Autodesk Inventor part; units mm, degrees
ref_plane "YZ Plane" through (0, 0, 0) normal (1, 0, 0) x (0, 1, 0)
ref_plane "XZ Plane" through (0, 0, 0) normal (0, 1, 0) x (-1, 0, 0)
ref_plane "XY Plane" through (0, 0, 0) normal (0, 0, 1) x (1, 0, 0)
sketch "スケッチ1" plane through (0, 0, 0) normal (0, 0, 1) x (1, 0, 0)
  circle A0 centre (0, 0) radius 21
  dimension "d0" = 42
extrude "押し出し1" add sketch "スケッチ1" along normal blind 5
sketch "スケッチ2" plane through (0, 0, 5) normal (0, 0, 1) x (1, 0, 0)
  circle A0 centre (0, 0) radius 14
  circle A1 centre (0, 0) radius 17.5
  circle A2 centre (0, 0) radius 21
  dimension "d3" = 28
  dimension "d8" = 7
  dimension "d9" = 3.5
extrude "押し出し3" add sketch "スケッチ2" along normal blind 5 contours A1
fillet "フィレット1" radius 1 4 edges at (-14, 0, 10) (-17.5, 0, 10) (-17.5, 0, 5) (-21, 0, 5)
extrude "押し出し4" add sketch "スケッチ2" along normal blind 4 contours A0
equation "\"d9\" = 0.5 * d8"
properties part number "inkpad"
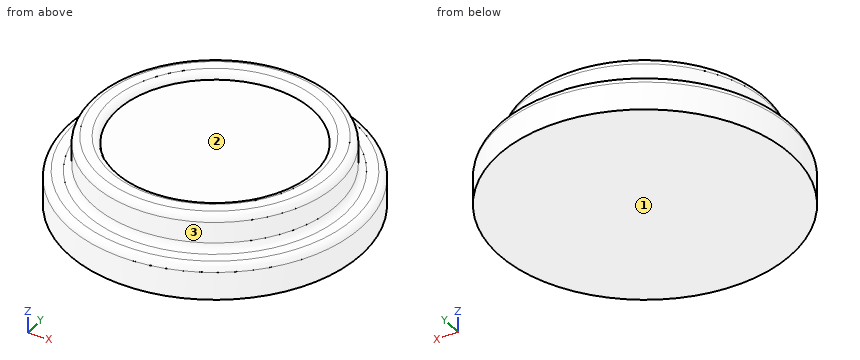
The listing builds one solid part. Answer for the finished solid, in the listing's coordinates (mm). Face numbers are marked on the shaded views. Round coordinates to 2 decimals unless told otherwise and drop trailing zeros. Loops run counter-clockwise (first coordinate to the right, second up) from the corner with the lowest first, then second, coordinate; pieces in that order, holes last. Notation, with made-up numbers: (-24, -15) -> (25, -15) arc R27 cw to (25, 16) -> close; hole circle Ø4 at (51, -13). An arc over 180 degrees is marked (long way). Use one line per item in the form item = value.
1. The part is cut by section C-C on z = 1.5. Determine the outline of the cut face in (x, y).
Answer key:
outline = circle Ø42 at (0, 0)
2. Find the intervals of material crossed by probe 1 along Z at (x, y) = (8, 2); probe 2 along Y at (x, z) = (-4.5, 6.75); probe 3 along X at (y, z) = (3.5, 7.5), in increasing order. Write a range as [from, to].
Answer key:
probe_1 = [0, 9]
probe_2 = [-16.91, 16.91]
probe_3 = [-17.15, 17.15]
3. For a pull along Y with two mould halves and no side action, classify the marked faces 1, 2 and 3 as released by +Y, released by -Y, zero draft, split by the parting line, or undercut.
Answer key:
face_1 = zero draft
face_2 = undercut
face_3 = split by the parting line
4. Flat-ended cylindrical pins translate along their axes: pin 1 Ø12 at (x, y) = (4, 0) entering from +Z; pin 2 Ø22.5 at (x, y) = (3.5, 0) entering from +Z; pin 3 Ø1.5 at (y, z) = (9.5, 3) entering from +X. Find the tip coordinate at first contact, or state that the pin passes through.
Answer key:
pin_1 = 9
pin_2 = 9.97
pin_3 = 19.09
5. The part is cut by section D-D on z = 7.5. Determine the outline of the cut face in (x, y).
Answer key:
outline = circle Ø35 at (0, 0)
6. The part is cut by section A-A on y = 0. Determine the outline of the cut face in (x, z).
Answer key:
outline = (-21, 0) -> (21, 0) -> (21, 4) arc R1 ccw to (20, 5) -> (18.5, 5) arc R1 cw to (17.5, 6) -> (17.5, 9) arc R1 ccw to (16.5, 10) -> (15, 10) arc R1 ccw to (14, 9) -> (-14, 9) arc R1 ccw to (-15, 10) -> (-16.5, 10) arc R1 ccw to (-17.5, 9) -> (-17.5, 6) arc R1 cw to (-18.5, 5) -> (-20, 5) arc R1 ccw to (-21, 4) -> close
